Geometry check sheet. Reference: the model listing, model coordinates, mm. Face numbers are marked on the shaded views. A direction names the side the tool comes from. Give positions to 0.01 mm unless a question says otherwise; leave off trailing zeros. Order: outer loops, then holes, each group sorted by start corner. A loop starts at its lowest first (then second) coordinate and runs counter-clockwise, first axis right, second up. Notation, with made-up numbers: (-20, -22) - (16, -22) arc R31 ccw to (16, 6) - close; hole circle Ø3 at (-30.5, 52.5). An arc over 180 degrees is marked (long way). Put each result on its own line as item: value. Start each with the question number.
```python
from build123d import *

# Parameters (mm, degrees)
F0_W     = 355.6
F0_H     = 406.4
F1_DEPTH = 76.2
F2_R     = 41.275
F3_DEPTH = 76.201
F4_W     = 257.175
F4_H     = 307.975
F5_DEPTH = 6.35


with BuildPart() as f1:
    # F0 (on Top) → F1 (new body)
    with BuildSketch(Plane.XY):
        Rectangle(F0_W, F0_H)
    extrude(amount=F1_DEPTH)

    # F2 (on face) → F3 (cut, through all)
    with BuildSketch(Plane.XY.offset(76.2)):
        Circle(F2_R)
    extrude(amount=-F3_DEPTH, mode=Mode.SUBTRACT)

    # F4 (on face) → F5 (cut)
    with BuildSketch(Plane.XY.offset(76.2)):
        Rectangle(F4_W, F4_H)
    extrude(amount=-F5_DEPTH, mode=Mode.SUBTRACT)


solid = f1.part
```
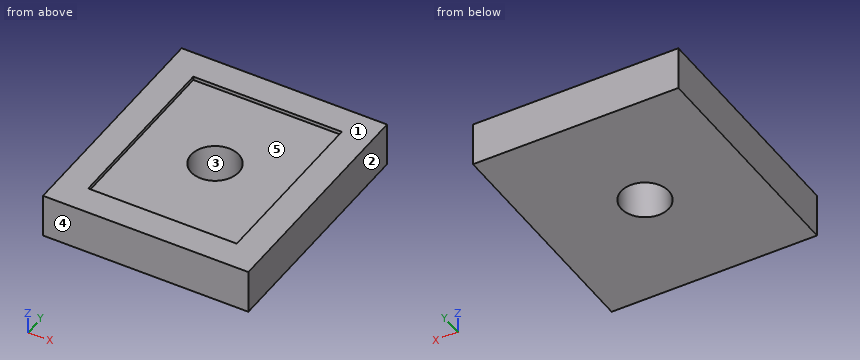
Item 1: Cross-section at C-C (z = 16). Enter the section's corners in (x, y) (3 decimals), and give its area (3 significant figures).
Item 2: Set-up check for the marked faces 4 and 5: record each of +Z, -Z, +X, -X, +Y, -Y from which the full face is reachable in a straight line by a thin tool's end or side.
Item 3: Gauge pin test, flat end, axial feed: pin 1 Ø1 at (x, y) = (129.5, -75.5) entering from -Z. Record the tip position at first contact, or that the pin passes through.
Item 4: Release check for a two-part mould opening along X. For the marked faces 1, 2 and 3 record: +X half, -X half, draft (parallel to the pull), parting line (faces both ways), or undercut.
Item 5: Cross-section at D-D (y = -145). Enter the section's corners in (x, z), and give its area (3 significant figures).
Item 6: Thickness scan on line 1 along Y through (x, z) = (0, 30) (3 decimals); line 2 along Y through (x, z) = (21, 41); line 3 along X through (y, z) = (-33, 20.5). Record the ranges inside material, lowest first.
Recorded:
1. outline: (-177.8, -203.2) - (177.8, -203.2) - (177.8, 203.2) - (-177.8, 203.2) - close; hole circle Ø82.55 at (0, 0)
1. area: 139,000 mm^2
2. face 4: +Z, -Z, +X, -X, -Y
2. face 5: +Z
3. pin 1: stops at z = 0
4. face 1: draft
4. face 2: +X half
4. face 3: undercut
5. outline: (-177.8, 0) - (177.8, 0) - (177.8, 76.2) - (128.59, 76.2) - (128.59, 69.85) - (-128.59, 69.85) - (-128.59, 76.2) - (-177.8, 76.2) - close
5. area: 25,500 mm^2
6. line 1: y = -203.2 to -41.275, 41.275 to 203.2
6. line 2: y = -203.2 to -35.53, 35.53 to 203.2
6. line 3: x = -177.8 to -24.79, 24.79 to 177.8
